Build history of the part. All positions in model axes, mm. Face numbers are marked on the shaded views. A direction names the side the tool comes from. Give positions to 0.01 mm unless a question says otherwise; leave off trailing zeros. Order: outer loops, then holes, each group sorted by start corner. A loop starts at its lowest first (then second) coordinate and runs counter-clockwise, first axis right, second up. Notation, with made-up numbers: (84, -31) - (102, -31) arc R14 cw to (102, -24) - close; hole circle Ø6 at (78, -26.5). An arc over 180 degrees is marked (long way). Answer in a Markdown table with one row per item.
```python
from build123d import *

# Parameters (mm, degrees)
SKETCH1_R           = 4
SKETCH1_R_2         = 1.25
BOSS_EXTRUDE1_DEPTH = 30
BOSS_EXTRUDE2_DEPTH = 12
SKETCH3_R           = 1
CUT_EXTRUDE1_DEPTH  = 12


with BuildPart() as part:
    # Sketch1 → Boss-Extrude1 (new body)
    with BuildSketch(Plane.XY):
        with Locations((0, 491.000207075)):
            Circle(SKETCH1_R)
        with Locations((0, 491.000207075)):
            Circle(SKETCH1_R_2, mode=Mode.SUBTRACT)
    extrude(amount=BOSS_EXTRUDE1_DEPTH)

    # Sketch2 → Boss-Extrude2 (add)
    with BuildSketch(Plane.XY.offset(30)):
        with BuildLine():
            Line((0.46875, 495.978185926), (16.328125, 494.484792271))
            ThreePointArc((16.328125, 494.484792271), (19.5, 491.000207075), (16.328125, 487.51562188))
            Line((16.328125, 487.51562188), (0.46875, 486.022228224))
            ThreePointArc((0.46875, 486.022228224), (-5, 491.000207075), (0.46875, 495.978185926))
        make_face()
    extrude(amount=-BOSS_EXTRUDE2_DEPTH)

    # Sketch3 → Cut-Extrude1 (cut)
    with BuildSketch(Plane.XY.offset(30)):
        with Locations((16, 491.000207075)):
            Circle(SKETCH3_R)
    extrude(amount=-CUT_EXTRUDE1_DEPTH, mode=Mode.SUBTRACT)


solid = part.part
```
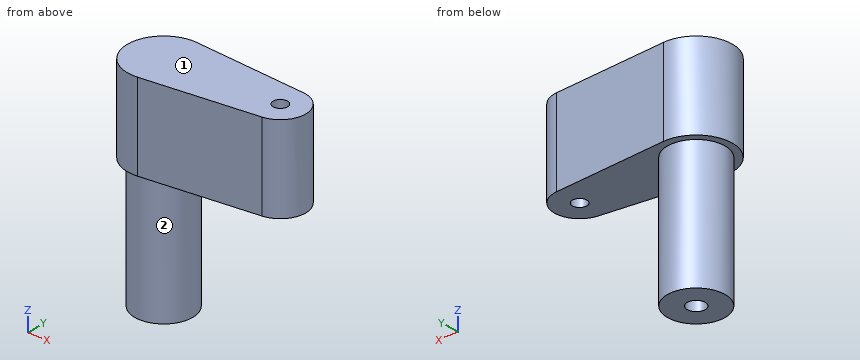
1. Cut at C-C on x = 0. Write the cut outline in (y, z), and give its area (3 significant figures).
Check result:
| item | result |
|---|---|
| outline | (486, 18) - (487, 18) - (487, 0) - (489.75, 0) - (489.75, 18) - (492.25, 18) - (492.25, 0) - (495, 0) - (495, 18) - (496, 18) - (496, 30) - (486, 30) - close |
| area | 219 mm² |
2. Cut at B-B on z = 26.5. Write the cut outline in (x, y), and give its area (3 significant figures).
Check result:
| item | result |
|---|---|
| outline | (0.47, 486.02) - (16.33, 487.52) arc R3.5 ccw to (16.33, 494.48) - (0.47, 495.98) arc R5 ccw (long way) to start; hole circle Ø2 at (16, 491) |
| area | 192 mm² |
3. Probe line 1 (Z direction, x = 1.25, y = 495.25); line 2 (Y direction, x = 0, z = 4); line 3 (Y direction, x = 16, z = 22.5). List the from-to ranges inside material, lowest first.
Check result:
| item | result |
|---|---|
| line 1 | z = 18 to 30 |
| line 2 | y = 487 to 489.75, 492.25 to 495 |
| line 3 | y = 487.48 to 490, 492 to 494.52 |
4. Cut at D-D on y = 488. Write the cut outline in (x, z), and give its area (3 significant figures).
Check result:
| item | result |
|---|---|
| outline | (-4, 18) - (-2.65, 18) - (-2.65, 0) - (2.65, 0) - (2.65, 18) - (17.8, 18) - (17.8, 30) - (-4, 30) - close |
| area | 357 mm² |
5. Which spindle directions (+Z, -Z, +X, -X, +Y, -Y) get a long thin tool onto all of the face, cutting with end or side? Do the marked faces 1 and 2. Say none if no direction does.
Check result:
| item | result |
|---|---|
| face 1 | +Z, +X, -X, +Y, -Y |
| face 2 | -Z |
6. Cut at A-A on x = 16. Write the cut outline in (y, z).
Check result:
| item | result |
|---|---|
| outline | (487.48, 18) - (490, 18) - (490, 30) - (487.48, 30) - close; (492, 18) - (494.52, 18) - (494.52, 30) - (492, 30) - close |
7. Drop flat-ended pins along their axis: P1, Ø1, axis at x = 9, y = 492, coming from the -Z side; P2, Ø2, axis at x = 0, y = 490.5, coming from the -Z side; P3, Ø3, axis at x = 13, z = 27, coming from the -Y side; P4, Ø4, axis at y = 495, z = 3.5, coming from the +X side. Give the stop position or say it passes through.
Check result:
| item | result |
|---|---|
| P1 | stops at z = 18 |
| P2 | stops at z = 0 |
| P3 | stops at y = 487.06 |
| P4 | stops at x = 3.46 |
